Design review of the part built by this model. Coordinates are the model's own, in mm. A direction names the side the tool comes from. Coordinates: 2 decimals unless noted, no trailing zeros. Write each loop counter-clockwise with the first axis right and the second up, starting at its lowest first coordinate (ties: lowest second). Pieces come first, ordered by that corner, then holes.
Q1. Machinability: for faces 4 (the face through (-1, -1, 0)), 5 (the face through (1, 0, -0.5)), 6 (the face through (-1.22, -0.27, -9.74)), which of the approach directions +Z, -Z, +X, -X, +Y, -Y give a long, thin tool a straight path to every point of the face, cutting with its end or side? Answer none if there is none.
Q2. The part is to be moulded in two halves that separate along Y. For faces 1 (the face through (0, 0, -16.5)), 2 (the face through (0.49, -0.87, -0.54)), 3 (the face through (2.23, -0.29, -1.31)), say which applies: +Y half, -Y half, draft (parallel to the pull), parting line (faces both ways), or undercut.
Q3. To check wall thickness, follow probe 1 along Z at (x, y) = (-0.5, -1.8); probe 2 along X at (y, z) = (-0.9, -13); probe 3 along X at (y, z) = (0.1, -9.5). State the ranges of each line that lie inside material, in increasing order.
Q4. Add section A-A, the plane z = -6.25. Give the boundary of the cut face in (x, y), plus the area to 3 significant figures.
Q5. Clearance check with a flat-ended pin moving along its axis: pin 1 Ø2 at (x, z) = (1, -12) entering from -Y. State where the tip first meets the part, or that it passes through.
from build123d import *

# Parameters (mm, degrees)
CUT_EXTRUDE1_DEPTH = 1.1


with BuildPart() as part:
    # Sketch1 → Revolve1 (revolve)
    with BuildSketch(Plane(origin=(0, 0, 0), x_dir=(0, 0, -1), z_dir=(1, 0, 0))):
        with BuildLine():
            Line((0, 0), (0, 2))
            Line((0, 2), (0.25, 2.25))
            Line((0.25, 2.25), (2.34, 2.25))
            Line((2.34, 2.25), (2.5, 2.09))
            Line((2.5, 2.09), (2.5, 1.55))
            ThreePointArc((2.5, 1.55), (2.515193643, 1.49701055), (2.556157637, 1.460123155))
            Line((2.556157637, 1.460123155), (2.966157637, 1.260123155))
            ThreePointArc((2.966157637, 1.260123155), (2.98750205, 1.25256365), (3.01, 1.25))
            Line((3.01, 1.25), (16.275, 1.25))
            Line((16.275, 1.25), (16.5, 1.025))
            Line((16.5, 1.025), (16.5, 0))
            Line((16.5, 0), (0, 0))
        make_face()
    revolve(axis=Axis((0, 0, 0), (0, 0, -1)))

    # Sketch2 → Cut-Extrude1 (cut)
    with BuildSketch(Plane.XY):
        Polygon((0, 1.154700538), (-1, 0.577350269), (-1, -0.577350269), (0, -1.154700538), (1, -0.577350269), (1, 0.577350269), align=None)
    extrude(amount=-CUT_EXTRUDE1_DEPTH, mode=Mode.SUBTRACT)

    # Sketch3 → Cut-Revolve2 (revolve, cut)
    with BuildSketch(Plane(origin=(0, 0, 0), x_dir=(0, 0, -1), z_dir=(1, 0, 0))):
        Polygon((1.1, 0), (1.1, 1), (1.677350269, 0), align=None)
    revolve(axis=Axis((0, 0, -1.1), (0, 0, -1)), mode=Mode.SUBTRACT)

    # Sketch4 → Cut-Revolve3 (revolve, cut)
    with BuildSketch(Plane(origin=(0, 0, 0), x_dir=(0, 0, -1), z_dir=(1, 0, 0))):
        Polygon((0, 1.154700538), (0, 1), (0.041451884, 1), align=None)
    revolve(axis=Axis((0, 0, 0), (0, 0, -1)), mode=Mode.SUBTRACT)


solid = part.part
Here are the results:
1. face 4: +Z, +X, -X, +Y, -Y
1. face 5: +Z
1. face 6: -Z
2. face 1: draft
2. face 2: undercut
2. face 3: parting line
3. probe 1: z = -2.5 to 0
3. probe 2: x = -0.87 to 0.87
3. probe 3: x = -1.25 to 1.25
4. outline: circle Ø2.5 at (0, 0)
4. area: 4.91 mm2
5. pin 1: stops at y = -1.25
